from build123d import *

# Parameters (mm, degrees)
SPUR_START             = -39.027193307
SPUR_GEAR_AI_OUTLINE_R = 1.5875
SPUR_GEAR_AI_DEPTH     = 9.525
SKETCH1_R              = 3.175
SKETCH1_R_2            = 1.5875
BOSS_EXTRUDE1_DEPTH    = 3.302


# Read off the part's stored shape, not the designer's step: spur gear_ai
with BuildPart() as part:
    # spur gear_ai outline → spur gear_ai (new body)
    with BuildSketch(Plane.YZ.offset(SPUR_START)):
        with BuildLine():
            ThreePointArc((11.105383233, 11.622198105), (11.20659768, 11.720869772), (11.305269347, 11.822084219))
            ThreePointArc((11.305269347, 11.822084219), (11.004316623, 12.744174963), (10.288347307, 13.398553922))
            ThreePointArc((10.288347307, 13.398553922), (10.533298325, 13.770131825), (10.732618719, 14.168054581))
            ThreePointArc((10.732618719, 14.168054581), (11.657312179, 13.875196444), (12.60634255, 14.075609112))
            ThreePointArc((12.60634255, 14.075609112), (12.644660999, 14.211668506), (12.679505946, 14.348658621))
            ThreePointArc((12.679505946, 14.348658621), (11.95782787, 14.996736269), (11.010590774, 15.205460412))
            ThreePointArc((11.010590774, 15.205460412), (11.036935627, 15.649731825), (11.010590774, 16.094003238))
            ThreePointArc((11.010590774, 16.094003238), (11.957827869, 16.302727382), (12.679505946, 16.950805029))
            ThreePointArc((12.679505946, 16.950805029), (12.644660999, 17.087795145), (12.60634255, 17.223854538))
            ThreePointArc((12.60634255, 17.223854538), (11.657312179, 17.424267206), (10.732618719, 17.131409069))
            ThreePointArc((10.732618719, 17.131409069), (10.533298325, 17.529331825), (10.288347307, 17.900909728))
            ThreePointArc((10.288347307, 17.900909728), (11.004316623, 18.555288687), (11.305269347, 19.477379431))
            ThreePointArc((11.305269347, 19.477379431), (11.20659768, 19.578593878), (11.105383233, 19.677265545))
            ThreePointArc((11.105383233, 19.677265545), (10.183292489, 19.376312821), (9.52891353, 18.660343505))
            ThreePointArc((9.52891353, 18.660343505), (9.157335627, 18.905294523), (8.759412871, 19.104614918))
            ThreePointArc((8.759412871, 19.104614918), (9.052271007, 20.029308378), (8.85185834, 20.978338749))
            ThreePointArc((8.85185834, 20.978338749), (8.715798946, 21.016657197), (8.57880883, 21.051502144))
            ThreePointArc((8.57880883, 21.051502144), (7.930731183, 20.329824068), (7.722007039, 19.382586973))
            ThreePointArc((7.722007039, 19.382586973), (7.277735627, 19.408931825), (6.833464214, 19.382586973))
            ThreePointArc((6.833464214, 19.382586973), (6.62474007, 20.329824068), (5.976662423, 21.051502144))
            ThreePointArc((5.976662423, 21.051502144), (5.839672308, 21.016657197), (5.703612914, 20.978338749))
            ThreePointArc((5.703612914, 20.978338749), (5.503200246, 20.029308378), (5.796058383, 19.104614918))
            ThreePointArc((5.796058383, 19.104614918), (5.398135627, 18.905294523), (5.026557723, 18.660343505))
            ThreePointArc((5.026557723, 18.660343505), (4.372178765, 19.376312821), (3.45008802, 19.677265545))
            ThreePointArc((3.45008802, 19.677265545), (3.348873574, 19.578593878), (3.250201907, 19.477379431))
            ThreePointArc((3.250201907, 19.477379431), (3.551154631, 18.555288687), (4.267123947, 17.900909728))
            ThreePointArc((4.267123947, 17.900909728), (4.022172929, 17.529331825), (3.822852534, 17.131409069))
            ThreePointArc((3.822852534, 17.131409069), (2.898159074, 17.424267206), (1.949128703, 17.223854538))
            ThreePointArc((1.949128703, 17.223854538), (1.910810254, 17.087795145), (1.875965308, 16.950805029))
            ThreePointArc((1.875965308, 16.950805029), (2.597643384, 16.302727382), (3.544880479, 16.094003238))
            ThreePointArc((3.544880479, 16.094003238), (3.518535627, 15.649731825), (3.544880479, 15.205460412))
            ThreePointArc((3.544880479, 15.205460412), (2.597643384, 14.996736269), (1.875965308, 14.348658621))
            ThreePointArc((1.875965308, 14.348658621), (1.910810254, 14.211668505), (1.949128703, 14.075609112))
            ThreePointArc((1.949128703, 14.075609112), (2.898159074, 13.875196444), (3.822852534, 14.168054581))
            ThreePointArc((3.822852534, 14.168054581), (4.022172929, 13.770131825), (4.267123947, 13.398553922))
            ThreePointArc((4.267123947, 13.398553922), (3.551154631, 12.744174963), (3.250201907, 11.822084219))
            ThreePointArc((3.250201907, 11.822084219), (3.348873574, 11.720869772), (3.45008802, 11.622198105))
            ThreePointArc((3.45008802, 11.622198105), (4.372178765, 11.923150829), (5.026557723, 12.639120145))
            ThreePointArc((5.026557723, 12.639120145), (5.398135627, 12.394169127), (5.796058383, 12.194848732))
            ThreePointArc((5.796058383, 12.194848732), (5.503200246, 11.270155272), (5.703612914, 10.321124901))
            ThreePointArc((5.703612914, 10.321124901), (5.839672308, 10.282806453), (5.976662423, 10.247961506))
            ThreePointArc((5.976662423, 10.247961506), (6.62474007, 10.969639583), (6.833464214, 11.916876678))
            ThreePointArc((6.833464214, 11.916876678), (7.277735627, 11.890531825), (7.722007039, 11.916876678))
            ThreePointArc((7.722007039, 11.916876678), (7.930731183, 10.969639583), (8.57880883, 10.247961506))
            ThreePointArc((8.57880883, 10.247961506), (8.715798946, 10.282806453), (8.85185834, 10.321124901))
            ThreePointArc((8.85185834, 10.321124901), (9.052271007, 11.270155272), (8.759412871, 12.194848732))
            ThreePointArc((8.759412871, 12.194848732), (9.157335627, 12.394169127), (9.52891353, 12.639120145))
            ThreePointArc((9.52891353, 12.639120145), (10.183292489, 11.923150829), (11.105383233, 11.622198105))
        make_face()
        with Locations((7.277735627, 15.649731825)):
            Circle(SPUR_GEAR_AI_OUTLINE_R, mode=Mode.SUBTRACT)
    extrude(amount=SPUR_GEAR_AI_DEPTH)

    # Sketch1 → Boss-Extrude1 (add)
    with BuildSketch(Plane(origin=(-29.502193307, 0, 0), x_dir=(0, 0, -1), z_dir=(1, 0, 0))):
        with Locations(Location((-15.649731825, 7.277735627, 0), (0, 0, 180))):
            Circle(SKETCH1_R)
        with Locations((-15.649731825, 7.277735627)):
            Circle(SKETCH1_R_2, mode=Mode.SUBTRACT)
    extrude(amount=BOSS_EXTRUDE1_DEPTH)


solid = part.part
Here's how the part is built. I have some questions about the finished solid (model axes, mm). Coordinates: 2 decimals unless noted, no trailing zeros. Loops run counter-clockwise (first coordinate to the right, second up) from the corner with the lowest first, then second, coordinate; pieces in that order, holes last.
1. Imagine slicing it at C-C, the plane z = 20. Please give me the cut outline in (x, y).
2. Imagine slicing it at B-B, the plane y = 12.25. Please give me the cut outline in (x, z), and give its area (3 significant figures).
3. Imagine slicing it at A-A, the plane z = 16.75. Please give me the cut outline in (x, y).
4. For P1, Ø6, axis at x = -34, z = 18, coming from the -Y side; P2, Ø1, axis at x = -28.5, y = 8, coming from the +Z side; P3, Ø1.5, axis at x = -31, y = 6, coming from the -Z side, each with a flat end and sliding along its axis, tell me the tip position at first contact or that it passes through.
5. I need wall thicknesses on L1, parallel to Y at x = -30, z = 12.25; L2, parallel to Y at x = -30, z = 19.5; L3, parallel to Z at x = -32.5, y = 3.75. Which ranges of each line are inside material? Lowest first, please.
6. Imagine slicing it at D-D, the plane y = 9.75. Please give me the cut outline in (x, z).
7. If we mould it in two halves opening along Y, with no side actions, what happens to faces 1 (the cylindrical face through (-34.331, 11.644, 13.876)), 2 (the cylindrical face through (-27.874, 10.377, 14.961))? For each: pulls with the +Y half, pulls with the -Y half, needs draft (parallel to the pull), parting line crosses it, or undercut.
Taken from the geometry:
1. outline: (-39.03, 5.5) - (-29.5, 5.5) - (-29.5, 6.76) - (-39.03, 6.76) - close; (-39.03, 7.8) - (-29.5, 7.8) - (-29.5, 9.05) - (-39.03, 9.05) - close
2. outline: (-39.03, 13.94) - (-29.5, 13.94) - (-29.5, 14.81) - (-39.03, 14.81) - close; (-39.03, 16.49) - (-29.5, 16.49) - (-29.5, 17.36) - (-39.03, 17.36) - close
2. area: 16.6 mm2
3. outline: (-39.03, 2.03) - (-29.5, 2.03) - (-29.5, 4.3) - (-26.2, 4.3) - (-26.2, 6.13) - (-39.03, 6.13) - close; (-39.03, 8.42) - (-26.2, 8.42) - (-26.2, 10.26) - (-29.5, 10.26) - (-29.5, 12.53) - (-39.03, 12.53) - close
4. P1: stops at y = 1.88
4. P2: stops at z = 18.82
4. P3: stops at z = 10.25
5. L1: y = 3.32 to 4.76, 5.67 to 8.88, 9.8 to 11.23
5. L2: y = 3.27 to 4.15, 5.61 to 6.83, 7.72 to 8.95, 10.41 to 11.28
5. L3: z = 11.66 to 13, 14.12 to 17.18, 18.3 to 19.64
6. outline: (-39.03, 12.31) - (-29.5, 12.31) - (-29.5, 13.66) - (-26.2, 13.66) - (-26.2, 17.64) - (-29.5, 17.64) - (-29.5, 18.99) - (-39.03, 18.99) - close
7. face 1: undercut
7. face 2: parting line crosses it
